```python
from build123d import *

# Parameters (mm, degrees)
SKETCH1_R                            = 2.0193
BOSS_EXTRUDE1_DEPTH                  = 69.8246
F_10_32_TAPPED_HOLE1_D               = 4.0386
F_10_32_TAPPED_HOLE1_DEPTH           = 16.34744
F_10_32_TAPPED_HOLE1_TIP             = 1.213317848
F_10_32_TAPPED_HOLE1_ON_FACE_2_D     = 4.0386
F_10_32_TAPPED_HOLE1_ON_FACE_2_DEPTH = 16.34744
F_10_32_TAPPED_HOLE1_ON_FACE_2_TIP   = 1.213317848
SKETCH3_R                            = 8.89
SKETCH3_R_2                          = 6.35
CUT_EXTRUDE_THIN1_DEPTH              = 7.9375


with BuildPart() as part:
    # Sketch1 → Boss-Extrude1 (new, symmetric)
    with BuildSketch(Plane(origin=(0, 0, 0), x_dir=(0, 0, -1), z_dir=(1, 0, 0))):
        with BuildLine():
            ThreePointArc((4.181770846, 5.456960429), (3.437499983, 5.953924622), (2.634980936, 6.35))
            Line((2.634980936, 6.35), (-2.634980936, 6.35))
            ThreePointArc((-2.634980936, 6.35), (-3.437499983, 5.953924622), (-4.181770846, 5.456960429))
            Line((-4.181770846, 5.456960429), (-6.816751782, 0.893039571))
            ThreePointArc((-6.816751782, 0.893039571), (-6.874999966, 0), (-6.816751782, -0.893039571))
            Line((-6.816751782, -0.893039571), (-4.181770846, -5.456960429))
            ThreePointArc((-4.181770846, -5.456960429), (-3.437499983, -5.953924622), (-2.634980936, -6.35))
            Line((-2.634980936, -6.35), (2.634980936, -6.35))
            ThreePointArc((2.634980936, -6.35), (3.437499983, -5.953924622), (4.181770846, -5.456960429))
            Line((4.181770846, -5.456960429), (6.816751782, -0.893039571))
            ThreePointArc((6.816751782, -0.893039571), (6.860422465, -0.447468582), (6.874999966, 0))
            ThreePointArc((6.874999966, 0), (6.860422465, 0.447468582), (6.816751782, 0.893039571))
            Line((6.816751782, 0.893039571), (4.181770846, 5.456960429))
        make_face()
        Circle(SKETCH1_R, mode=Mode.SUBTRACT)
    extrude(amount=BOSS_EXTRUDE1_DEPTH, both=True)

    # #10-32 Tapped Hole1
    with Locations(Plane(origin=(69.8246, 0, 0), x_dir=(0, 0, 1), z_dir=(1, 0, 0))):
        with Locations((0, 0)):
            Hole(F_10_32_TAPPED_HOLE1_D / 2, depth=F_10_32_TAPPED_HOLE1_DEPTH)
            with Locations((0, 0, -(F_10_32_TAPPED_HOLE1_DEPTH + F_10_32_TAPPED_HOLE1_TIP / 2))):  # 118° drill point
                Cone(0, F_10_32_TAPPED_HOLE1_D / 2, F_10_32_TAPPED_HOLE1_TIP, mode=Mode.SUBTRACT)

    # #10-32 Tapped Hole1 on face 2
    with Locations(Plane(origin=(-69.8246, 0, 0), x_dir=(0, 0, 1), z_dir=(1, 0, 0))):
        with Locations((0, 0)):
            Hole(F_10_32_TAPPED_HOLE1_ON_FACE_2_D / 2, depth=F_10_32_TAPPED_HOLE1_ON_FACE_2_DEPTH)
            with Locations((0, 0, -(F_10_32_TAPPED_HOLE1_ON_FACE_2_DEPTH + F_10_32_TAPPED_HOLE1_ON_FACE_2_TIP / 2))):  # 118° drill point
                Cone(0, F_10_32_TAPPED_HOLE1_ON_FACE_2_D / 2, F_10_32_TAPPED_HOLE1_ON_FACE_2_TIP, mode=Mode.SUBTRACT)

    # Sketch3 → Cut-Extrude-Thin1 (cut)
    with BuildSketch(Plane(origin=(69.8246, 0, 0), x_dir=(0, 0, -1), z_dir=(1, 0, 0))):
        Circle(SKETCH3_R)
        Circle(SKETCH3_R_2, mode=Mode.SUBTRACT)
    extrude(amount=-CUT_EXTRUDE_THIN1_DEPTH, mode=Mode.SUBTRACT)


solid = part.part
```
Can you work these out from the model? Positions are in its coordinate system, mm. A direction names the side the tool comes from. Give positions to 0.01 mm unless a question says otherwise; leave off trailing zeros. Loops run counter-clockwise (first coordinate to the right, second up) from the corner with the lowest first, then second, coordinate; pieces in that order, holes last. Notation, with made-up numbers: M -35,48 L 17,48 A13 cw 17,60 Z; hole C 11.5,56.5 d4. An arc over 180 degrees is marked long. Answer in a Markdown table with one row per item.
1. Which directions (+Z, -Z, +X, -X, +Y, -Y) give clear straight access to the entire face, cutting with the end or side of a thin tool? Please do faces 1 (the flat face through (61.887, 6, -3)), 2 (the flat face through (61.887, 6, 3)), 3 (the flat face through (-3.05, -3.14, 5.52)), 4 (the flat face through (61.887, -6, -3)), 5 (the cylindrical face through (65.91, -6.2, 1.38)).
Taken from the geometry:
| item | result |
|---|---|
| face 1 | -Z, +X, +Y |
| face 2 | +Z, +X, +Y |
| face 3 | +Z, +X, -X, -Y |
| face 4 | -Z, +X, -Y |
| face 5 | +X |
2. For pin 1 Ø3 at (x, y) = (22, -0.5) entering from -Z (3 decimals); pin 2 Ø3 at (x, z) = (25, 4.5) entering from +Y; pin 3 Ø2 at (x, y) = (-1, -3.5) entering from -Z; pin 4 Ø3 at (y, z) = (0, 0) entering from -X, each with a flat end and sliding along its axis, tell me the tip position at first contact or that it passes through.
Taken from the geometry:
| item | result |
|---|---|
| pin 1 | stops at z = -6.875 |
| pin 2 | stops at y = 6.19 |
| pin 3 | stops at z = -5.89 |
| pin 4 | passes through |
3. Thinking about a two-plate mould opening in Y: for faces 6 (the cylindrical face through (-0.978, 0.607, -1.926)), 7 (the flat face through (61.887, -6, 3)), 8 (the flat face through (-5, -6.35, 0)), which applies, released by +Y, released by -Y, zero draft, split by the parting line, or undercut?
Taken from the geometry:
| item | result |
|---|---|
| face 6 | undercut |
| face 7 | zero draft |
| face 8 | released by -Y |
4. If I drill on line 1 along Y through (x, z) = (4, 0); line 2 along Z through (x, y) = (53.5, 0.25); line 3 along Z through (x, y) = (-48, 3.25), over which ranges is the centre line in solid material (lowest first)?
Taken from the geometry:
| item | result |
|---|---|
| line 1 | y = -6.35 to -2.02, 2.02 to 6.35 |
| line 2 | z = -6.87 to -2, 2 to 6.87 |
| line 3 | z = -5.46 to 5.46 |
5. Suppose I cut it at A-A on x = 28. Write out the boundary of the cut face in (y, z) (3 decimals), plus the area to 3 significant figures.
Taken from the geometry:
| item | result |
|---|---|
| outline | M -6.35,-2.635 A6.875 ccw -5.457,-4.182 L -0.893,-6.817 A6.875 ccw 0.893,-6.817 L 5.457,-4.182 A6.875 ccw 6.35,-2.635 L 6.35,2.635 A6.875 ccw 5.457,4.182 L 0.893,6.817 A6.875 ccw -0.893,6.817 L -5.457,4.182 A6.875 ccw -6.35,2.635 Z; hole C 0,0 d4.039 |
| area | 125 mm² |
